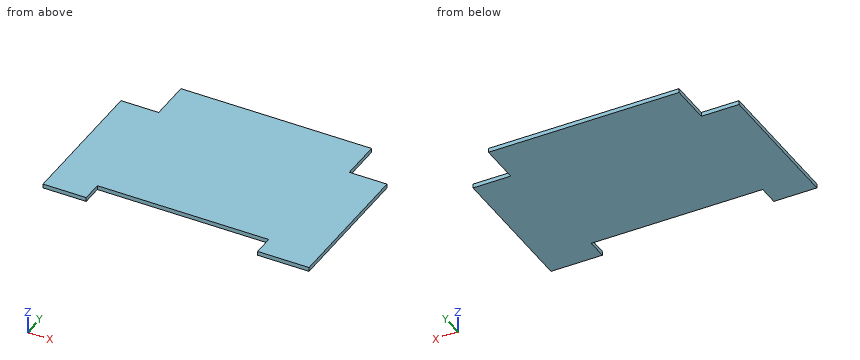
from build123d import *

# Parameters (mm, degrees)
SKETCH1_W           = 388
SKETCH1_H           = 270
BOSS_EXTRUDE1_DEPTH = 6
SKETCH2_W           = 55
SKETCH2_H           = 60
CUT_EXTRUDE1_DEPTH  = 40
SKETCH3_W           = 250
SKETCH3_H           = 30
CUT_EXTRUDE2_DEPTH  = 10


with BuildPart() as part:
    # Sketch1 → Boss-Extrude1 (new body)
    with BuildSketch(Plane.XY):
        with Locations((83.131383381, 125.666802076)):
            Rectangle(SKETCH1_W, SKETCH1_H)
    extrude(amount=BOSS_EXTRUDE1_DEPTH)

    # Sketch2 → Cut-Extrude1 (cut)
    with BuildSketch(Plane(origin=(0, 0, 0), x_dir=(-1, 0, 0), z_dir=(0, 0, -1))):
        with Locations((-249.631383381, 230.666802076)):
            Rectangle(SKETCH2_W, SKETCH2_H)
        with Locations((83.368616619, 230.666802076)):
            Rectangle(SKETCH2_W, SKETCH2_H)
    extrude(amount=-CUT_EXTRUDE1_DEPTH, mode=Mode.SUBTRACT)

    # Sketch3 → Cut-Extrude2 (cut)
    with BuildSketch(Plane(origin=(0, 0, 0), x_dir=(-1, 0, 0), z_dir=(0, 0, -1))):
        with Locations((-77.131383381, 5.666802076)):
            Rectangle(SKETCH3_W, SKETCH3_H)
    extrude(amount=-CUT_EXTRUDE2_DEPTH, mode=Mode.SUBTRACT)


solid = part.part
The listing builds one solid part. Answer for the finished solid, in the listing's coordinates (mm). Coordinates: 2 decimals unless noted, no trailing zeros. Loops run counter-clockwise (first coordinate to the right, second up) from the corner with the lowest first, then second, coordinate; pieces in that order, holes last.
1) Flat-ended cylindrical pins translate along their axes: pin 1 Ø1.8 at (y, z) = (223.5, 3) entering from +X; pin 2 Ø1.8 at (x, z) = (115.5, 2.5) entering from -Y; pin 3 Ø3 at (x, z) = (260, 1.5) entering from +Y. Find the tip coordinate at first contact, or state that the pin passes through.
2) Find the intervals of material crossed by L1, parallel to X at y = 9, z = 3.55; L2, parallel to Y at x = 5.5, z = 0.75; L3, parallel to X at y = 214, z = 4.7, in increasing order.
3) Find section B-B on x = 197. Write down the section's boundary in (y, z).
4) Find section A-A on z = 3.7. Write down the section's boundary in (x, y), then the cut area to 3 significant figures.
Values:
1. pin 1: stops at x = 222.13
1. pin 2: stops at y = 20.67
1. pin 3: stops at y = 200.67
2. L1: x = -110.87 to -47.87, 202.13 to 277.13
2. L2: y = 20.67 to 260.67
2. L3: x = -55.87 to 222.13
3. outline: (20.67, 0) - (260.67, 0) - (260.67, 6) - (20.67, 6) - close
4. outline: (-110.87, -9.33) - (-47.87, -9.33) - (-47.87, 20.67) - (202.13, 20.67) - (202.13, -9.33) - (277.13, -9.33) - (277.13, 200.67) - (222.13, 200.67) - (222.13, 260.67) - (-55.87, 260.67) - (-55.87, 200.67) - (-110.87, 200.67) - close
4. area: 90,700 mm2
